The figure shows three views and two pictorial views of one solid part (mm, origin at its lowest corner). Answer the questions. A direction names the side the tool comes from. Round coordinates to 2 decimals unless told otherwise and drop trailing zeros. Order: outer loops, then holes, each group sorted by start corner. A loop starts at its lowest first (then second) coordinate and runs counter-clockwise, first axis right, second up. Notation, with made-up numbers: M 8,83.25 L 34,83.25 A29 ccw 34,112.25 Z; hole C -39.5,61 d11. An arc over 180 degrees is marked long. Return JSON: item names as keys, results as strings.
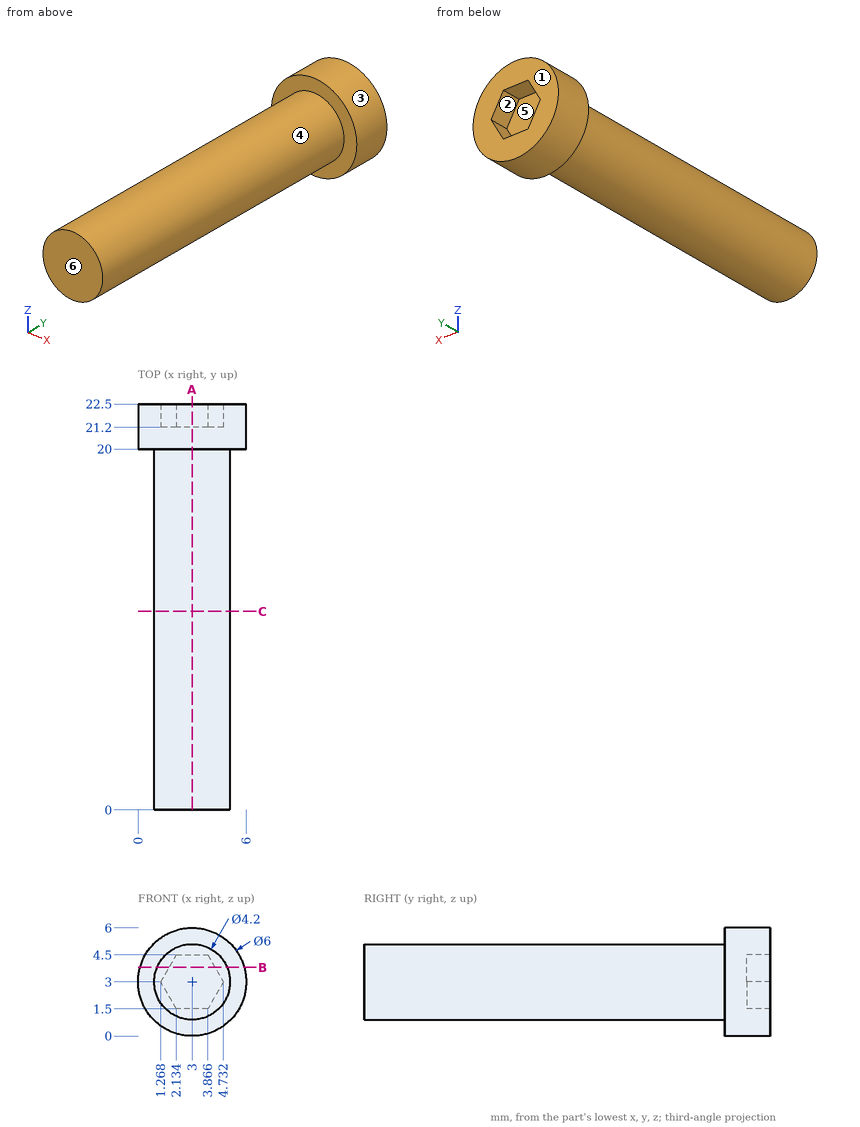
Item 1: Find section A-A (x = 3). Determine the outline of the cut face in (y, z), plus the area to 3 significant figures.
Output:
{"outline": "M 0,0.9 L 20,0.9 L 20,0 L 22.5,0 L 22.5,1.5 L 21.2,1.5 L 21.2,4.5 L 22.5,4.5 L 22.5,6 L 20,6 L 20,5.1 L 0,5.1 Z", "area": "95.1 mm^2"}
Item 2: Which of the six approach directions +Z, -Z, +X, -X, +Y, -Y give full straight-line access (tool end or side, diameter ignored) to the marked faces 4, 5 and 6?
Output:
{"face 4": "-Y", "face 5": "+Y", "face 6": "+Z, -Z, +X, -X, -Y"}
Item 3: The mould has two halves that part along X. Classify the marked faces 1, 2 and 3: pulls with the +X half, pulls with the -X half, needs draft (parallel to the pull), parting line crosses it, or undercut.
Output:
{"face 1": "needs draft", "face 2": "undercut", "face 3": "parting line crosses it"}
Item 4: Find section B-B (z = 3.8). Determine the outline of the cut face in (x, y), plus the area to 3 significant figures.
Output:
{"outline": "M 0.11,20 L 1.06,20 L 1.06,0 L 4.94,0 L 4.94,20 L 5.89,20 L 5.89,22.5 L 4.27,22.5 L 4.27,21.2 L 1.73,21.2 L 1.73,22.5 L 0.11,22.5 Z", "area": "88.8 mm^2"}
Item 5: Find section C-C (y = 11). Determine the outline of the cut face in (x, z), plus the area to 3 significant figures.
Output:
{"outline": "C 3,3 d4.2", "area": "13.9 mm^2"}
Item 6: Consider line 1 along Y through (x, z) = (4.2, 5.4); line 2 along Y through (x, z) = (2.85, 1.95); line 3 along Z through (x, y) = (1.6, 21.5) (1 decimal). Determine where each line is inside the solid, lowest interval first. Write a range as [from, to].
Output:
{"line 1": "y = [20, 22.5]", "line 2": "y = [0, 21.2]", "line 3": "z = [0.3, 2.4], [3.6, 5.7]"}
Item 7: Each of these flat-tipped pins is pushed along its axis until it touches: pin 1 (2 mm diameter, centred on y = 4, z = 4, fed in from +X); pin 2 (2 mm diameter, centred on x = 1.5, y = 3.5, fed in from +Z); pin 3 (1.5 mm diameter, centred on x = 1, y = 6.5, fed in from +Z). Where does it stop, or does it pass through?
Output:
{"pin 1": "stops at x = 5.1", "pin 2": "stops at z = 5.04", "pin 3": "stops at z = 4.69"}
